```python
from build123d import *


with BuildPart() as f1:
    # F0 (on Front) → F1 (revolve)
    with BuildSketch(Plane.XZ):
        with BuildLine():
            Line((0, 54.801697), (0, 55.376381))
            Line((0, 55.376381), (-3.544281, 55.376381))
            ThreePointArc((-3.544281, 55.376381), (-1.795285, 54.9463), (0, 54.801697))
        make_face()
        with BuildLine():
            Line((-3.544281, 55.376381), (0, 55.376381))
            Line((0, 55.376381), (0, 77.235242))
            ThreePointArc((0, 77.235242), (-11.072169, 67.813754), (-3.544281, 55.376381))
        make_face()
        with BuildLine():
            ThreePointArc((0, 54.801697), (-1.795285, 54.9463), (-3.544281, 55.376381))
            Line((-3.544281, 55.376381), (-5.688893, 55.376381))
            Line((-5.688893, 55.376381), (-44.340517, 55.376381))
            Line((-44.340517, 55.376381), (-44.340517, 45.523312))
            Line((-44.340517, 45.523312), (-6.700345, 45.523312))
            Line((-6.700345, 45.523312), (-6.700345, 30.348621))
            Line((-6.700345, 30.348621), (-5.688893, 30.348621))
            Line((-5.688893, 30.348621), (0, 30.348621))
            Line((0, 30.348621), (0, 54.801697))
        make_face()
        Polygon((0, 18.524483), (0, 30.348621), (-5.688893, 30.348621), (-14.780172, -16.947931), (-1.77362, -16.947931), align=None)
    revolve(axis=Axis((0, 0, 47.879862), (0, 0, -1)))


solid = f1.part
```
For this review, take the finished solid that the model builds, in its own axes (mm). A direction names the side the tool comes from. Round coordinates to 2 decimals unless told otherwise and drop trailing zeros. Write each loop counter-clockwise with the first axis right and the second up, starting at its lowest first coordinate (ties: lowest second). Pieces come first, ordered by that corner, then holes. Notation, with made-up numbers: (59, -11.5) -> (107, -11.5) arc R21 ccw to (107, 26.5) -> close; hole circle Ø8 at (21, 12). An arc over 180 degrees is marked (long way). Use one line per item in the form item = value.
1) Take a section at B-B, the plane y = -8. Count the separate pieces of the cut face and the enclosed holes in it, and give its area (3 significant figures).
Found:
separate_pieces = 3
enclosed_holes = 0
area = 1,600 mm2
2) Take a section at D-D, the plane y = -39. Write out the cut boundary in (x, z), and give its area (3 significant figures).
Found:
outline = (-21.1, 45.52) -> (21.1, 45.52) -> (21.1, 55.38) -> (-21.1, 55.38) -> close
area = 416 mm2
3) Mouldability with a two-part tool opening along Y and no side actions: class faces 3 (the conical face through (-9.823, 3.093, 6.369)), 4 (the flat face through (9, 1, 55.376)), 5 (the conical face through (0.19, -0.854, 1.037)) as +Y half, -Y half, draft (parallel to the pull), parting line (faces both ways), or undercut.
Found:
face_3 = parting line
face_4 = draft
face_5 = undercut
4) Take a section at C-C, the plane x = -19.5. Write out the cut boundary in (y, z), and give its area (3 significant figures).
Found:
outline = (-39.82, 45.52) -> (39.82, 45.52) -> (39.82, 55.38) -> (-39.82, 55.38) -> close
area = 785 mm2
5) Clearance check with flat-ended pins moving along their axes: pin 1 (3 mm diameter, centred on x = -2, y = 6.5, fed in from +Z); pin 2 (12 mm diameter, centred on x = -14, y = -20, fed in from -Z); pin 3 (1 mm diameter, centred on x = -29.5, y = -6, fed in from +Z). State where each tip first meets the part, or that it passes through.
Found:
pin_1 = 75.9
pin_2 = 45.52
pin_3 = 55.38
6) Take a section at A-A, the plane z = 36. Write out the cut boundary in (x, y), and give its area (3 significant figures).
Found:
outline = circle Ø13.4 at (0, 0)
area = 141 mm2
7) To check wall thickness, follow L1, parallel to Z at x = 0, y = 31; L2, parallel to X at y = 1, z = 47.5; L3, parallel to Y at x = 9.5, z = 47. State the ranges of each line that lie inside material, in increasing order. Write a range as from..to.
Found:
L1 = 45.52..55.38
L2 = -44.33..44.33
L3 = -43.31..43.31
8) Tool access review of faces 1 (the cylindrical face through (6.694, 0.295, 37.83)), 2 (the cylindrical face through (9.612, -43.286, 50.381)): name each direction out of +Z, -Z, +X, -X, +Y, -Y from which nothing blocks a thin tool from reaching the whole face with its end or side.
Found:
face_1 = none
face_2 = +Z, -Z
